Here's how the part is built. I have some questions about the finished solid (model axes, mm). Face numbers are marked on the shaded views. A direction names the side the tool comes from. Give positions to 0.01 mm unless a question says otherwise; leave off trailing zeros. Order: outer loops, then holes, each group sorted by start corner. A loop starts at its lowest first (then second) coordinate and runs counter-clockwise, first axis right, second up. Notation, with made-up numbers: M 85,2.5 L 130,2.5 A36 cw 130,38.5 Z; hole C 45.5,72 d3. An arc over 180 degrees is marked long. Use one line per item in the form item = value.
Autodesk Fusion 360 part; units mm, degrees
sketch "Sketch1" plane through (0, 0, 0) normal (0, 0, 1) x (1, 0, 0)
  line L0 (16.3, 9) -> (-16.3, 9) construction
  line L1 (-16.3, 9) -> (-16.3, -9) construction
  line L2 (-16.3, -9) -> (16.3, -9) construction
  line L3 (16.3, -9) -> (16.3, 9) construction
  line L4 (16.3, 9) -> (-16.3, -9) construction
  line L5 (-16.3, 9) -> (16.3, -9) construction
  line L6 (-8.6, 8) -> (13.7, 8)
  line L7 (13.7, 8) -> (13.7, -5.4)
  line L8 (13.7, -5.4) -> (-8.6, -5.4)
  line L9 (-8.6, -5.4) -> (-8.6, 8)
  circle A0 centre (0, 0) radius 3.5
  line L10 (2.4, -0.6) -> (-2.4, -0.6)
  line L11 (-2.4, -0.6) -> (-2.4, 0.6)
  line L12 (-2.4, 0.6) -> (2.4, 0.6)
  line L13 (2.4, 0.6) -> (2.4, -0.6)
  line L14 (2.4, -0.6) -> (-2.4, 0.6) construction
  line L15 (-2.4, -0.6) -> (2.4, 0.6) construction
  line L16 (0.6, -2.4) -> (-0.6, -2.4)
  line L17 (-0.6, -2.4) -> (-0.6, 2.4)
  line L18 (-0.6, 2.4) -> (0.6, 2.4)
  line L19 (0.6, 2.4) -> (0.6, -2.4)
  line L20 (0.6, -2.4) -> (-0.6, 2.4) construction
  line L21 (-0.6, -2.4) -> (0.6, 2.4) construction
  line L22 (-0.6, 2.4) -> (-2.5475, 2.4)
  line L23 (0.6, 2.4) -> (2.5475, 2.4)
  line L24 (-0.6, -2.4) -> (-2.5475, -2.4)
  line L25 (0.6, -2.4) -> (2.5475, -2.4)
  dimension "d1" = 32.6
  dimension "d2" = 18
  dimension "d3" = 3.6
  dimension "d4" = 1
  dimension "d5" = 2.6
  dimension "d6" = 7.7
  dimension "d7" = 7
  dimension "d8" = 4.8
  dimension "d9" = 1.2
  dimension "d10" = 1.2
  dimension "d11" = 4.8
extrude "Extrude1" add sketch "Sketch1" along normal blind 0.6 contours L6 L7 L8 L9 | A0 L10 L12 L13 L19 L23 L25 | A0 L18 L22 L23 | A0 L16 L24 L25 | A0 L10 L11 L12 L17 L22 L24 | L12 L17 L18 L19 | L10 L16 L17 L19 | L10 L12 L17 L19 | L10 L12 L13 L19 | L10 L11 L12 L17
extrude "Extrude2" add sketch "Sketch1" along normal blind 4 contours A0 L10 L12 L13 L19 L23 L25 | A0 L10 L11 L12 L17 L22 L24
fillet "Fillet1" radius 1 6 edges at (-1.5738, -2.4, 0.6) (-3.5, 0, 0.6) (1.5738, -2.4, 0.6) (3.5, 0, 0.6) (1.5738, 2.4, 0.6) (-1.5738, 2.4, 0.6)
fillet "Fillet1" radius 0.5 4 edges at (13.7, 8, 0.3) (-8.6, 8, 0.3) (13.7, -5.4, 0.3) (-8.6, -5.4, 0.3)
chamfer "Chamfer1" distance 0.4 angle 45 20 edges at (-8.4536, 7.8536, 0) (2.55, 8, 0) (13.5536, 7.8536, 0) (13.7, 1.3, 0) (13.5536, -5.2536, 0) (2.55, -5.4, 0) (-8.4536, -5.2536, 0) (-8.6, 1.3, 0) (-0.6, 1.5, 4) (-1.5, 0.6, 4) (-2.4, 0, 4) (-1.5, -0.6, 4) (-0.6, -1.5, 4) (0.6, -1.5, 4) (1.5, -0.6, 4) (2.4, 0, 4) (1.5, 0.6, 4) (0.6, 1.5, 4) (3.5, 0, 4) (-3.5, 0, 4)
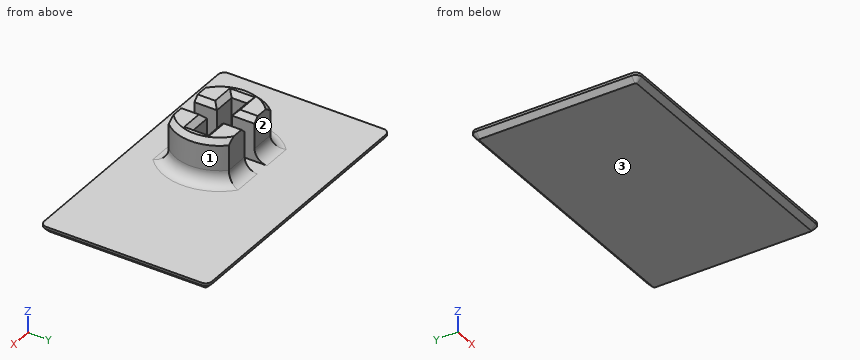
Q1. I need wall thicknesses on L1, parallel to Y at x = 0.75, z = 3.45; L2, parallel to Z at x = -7, y = 3.75; L3, parallel to X at y = 2.5, z = 0.9. Which ranges of each line are inside material? Lowest first, please.
Found:
L1 = -2.4 to -0.6, 0.6 to 2.4
L2 = 0 to 0.6
L3 = -2.84 to -0.6, 0.6 to 2.84
Q2. I want a section at A-A on z = 1.95. Write out the boundary of the cut face in (x, y), then the cut area to 3 significant figures.
Found:
outline = M -2.55,-2.4 L -0.6,-2.4 L -0.6,-0.6 L -2.4,-0.6 L -2.4,0.6 L -0.6,0.6 L -0.6,2.4 L -2.55,2.4 A3.5 ccw Z; M 0.6,-2.4 L 2.55,-2.4 A3.5 ccw 2.55,2.4 L 0.6,2.4 L 0.6,0.6 L 2.4,0.6 L 2.4,-0.6 L 0.6,-0.6 Z
area = 20.7 mm²
Q3. I'm going to push flat-ended pins straight in: pin 1 Ø1.6 at (x, z) = (2, 3) entering from +Y; pin 2 Ø1 at (y, z) = (0.5, 1.5) entering from +X; pin 3 Ø0.6 at (x, z) = (2, 2.5) entering from -Y; pin 4 Ø1 at (x, z) = (8.5, 3) entering from -Y. Where does each tip first touch, or does it pass through?
Found:
pin_1 = 2.4
pin_2 = 3.67
pin_3 = -2.4
pin_4 = through
Q4. I want a section at B-B on x = -6.5. Write out the boundary of the cut face in (y, z), then the cut area to 3 significant figures.
Found:
outline = M -5.4,0.4 L -5,0 L 7.6,0 L 8,0.4 L 8,0.6 L -5.4,0.6 Z
area = 7.88 mm²
Q5. On a 3-axis mill with a long thin cutter (end or side, diameter ignored), from which of +Z, -Z, +X, -X, +Y, -Y can I reach the whole of each face in a straight line? I mean the marked faces 1, 2 and 3. Say none if no direction works.
Found:
face_1 = +Z, +X
face_2 = +Z, +X, -X, +Y
face_3 = -Z, +X, -X, +Y, -Y
Q6. I want a section at C-C on y = 6.75. Write out the boundary of the cut face in (x, z), then the cut area to 3 significant figures.
Found:
outline = M -8.6,0.4 L -8.2,0 L 13.3,0 L 13.7,0.4 L 13.7,0.6 L -8.6,0.6 Z
area = 13.2 mm²
